```python
from build123d import *

# Parameters (mm, degrees)
SALIENTE_EXTRUIR2_DEPTH = 4
CORTAR_EXTRUIR1_DEPTH   = 4


with BuildPart() as part:
    # Croquis1 → Saliente-Extruir2 (new body)
    with BuildSketch(Plane(origin=(0, 0, 0), x_dir=(0, 0, -1), z_dir=(1, 0, 0))):
        Polygon((0, 0), (28.190778624, 10.2606043), (93.930174324, 76), (185, 76), (185, 6), (50, 6), (50, 0), align=None)
    extrude(amount=SALIENTE_EXTRUIR2_DEPTH)

    # Croquis2 → Cortar-Extruir1 (cut)
    with BuildSketch(Plane(origin=(4, 0, 0), x_dir=(0, 0, -1), z_dir=(1, 0, 0))):
        with BuildLine():
            Line((105, 6), (165, 6))
            Line((165, 6), (165, 26))
            ThreePointArc((165, 26), (135, 56), (105, 26))
            Line((105, 26), (105, 6))
        make_face()
    extrude(amount=-CORTAR_EXTRUIR1_DEPTH, mode=Mode.SUBTRACT)


solid = part.part
```
Verification items for the finished model (mm, model axes). A direction names the side the tool comes from. Round coordinates to 2 decimals unless told otherwise and drop trailing zeros. Loops run counter-clockwise (first coordinate to the right, second up) from the corner with the lowest first, then second, coordinate; pieces in that order, holes last. Notation, with made-up numbers: (71.25, 77) -> (81.25, 77) arc R31 cw to (81.25, 105) -> close; hole circle Ø10 at (59, 33.25). An arc over 180 degrees is marked (long way). Answer as a JSON object with one key per item and string values.
Q1. Scan lines: line 1 (Z direction, x = 0.7, y = 46); line 2 (Z direction, x = 1.75, y = 41.5); line 3 (Y direction, x = 0.7, z = -96). Record each from-to range of solid material in increasing order. Write a range as from..to.
Data:
{"line 1": "z = -185..-157.36, -112.64..-63.93", "line 2": "z = -185..-160.69, -109.31..-59.43", "line 3": "y = 6..76"}
Q2. Section check B-B (x = 3.3). Record the boundary of the cut face in (y, z).
Data:
{"outline": "(0, -50) -> (6, -50) -> (6, -105) -> (26, -105) arc R30 cw to (26, -165) -> (6, -165) -> (6, -185) -> (76, -185) -> (76, -93.93) -> (10.26, -28.19) -> (0, 0) -> close"}
Q3. Draft check along Z on faces 1 (the flat face through (4, 55, -114)), 2 (the flat face through (2, 16, -105)), 3 (the flat face through (2, 41, -185)), 4 (the flat face through (1.97, 5.06, -13.9)). Enter one of: pulls with the +Z half, pulls with the -Z half, needs draft (parallel to the pull), parting line crosses it, or undercut.
Data:
{"face 1": "needs draft", "face 2": "undercut", "face 3": "pulls with the -Z half", "face 4": "pulls with the +Z half"}
Q4. Section check D-D (z = -135). Record the boundary of the cut face in (x, y), then the cut area to 3 significant figures.
Data:
{"outline": "(0, 56) -> (4, 56) -> (4, 76) -> (0, 76) -> close", "area": "80.0 mm2"}
Q5. Go/stop test with flat-tipped pins: P1, Ø2, axis at x = 3, z = -173.5, coming from the -Y side; P2, Ø1.2, axis at x = 1.5, y = 12, coming from the +Z side. Record where each tip stops, or that it passes through.
Data:
{"P1": "stops at y = 6", "P2": "stops at z = -29.33"}
Q6. Section check C-C (z = -102). Record the boundary of the cut face in (x, y), then the cut area to 3 significant figures.
Data:
{"outline": "(0, 6) -> (4, 6) -> (4, 76) -> (0, 76) -> close", "area": "280 mm2"}
Q7. Access from +Z, -Z, +X, -X, +Y, -Y to the whole of each face (thin tool, end or side, straight path). Record for faces 5 (the flat face through (2, 3, -50)), 6 (the flat face through (2, 16, -165)), 7 (the flat face through (2, 0, -25)).
Data:
{"face 5": "-Z, +X, -X, -Y", "face 6": "+X, -X, -Y", "face 7": "+Z, -Z, +X, -X, -Y"}
Q8. Section check A-A (y = 47). Record the boundary of the cut face in (x, z), then the cut area to 3 significant figures.
Data:
{"outline": "(0, -185) -> (4, -185) -> (4, -156.42) -> (0, -156.42) -> close; (0, -113.58) -> (4, -113.58) -> (4, -64.93) -> (0, -64.93) -> close", "area": "309 mm2"}
